Part print with two shaded views. Sizes in mm from the minimum x, y, z corner. A direction names the side the tool comes from. Give positions to 0.01 mm unless a question says otherwise; leave off trailing zeros. Write each loop counter-clockwise with the first axis right and the second up, starting at its lowest first coordinate (ties: lowest second). Pieces come first, ordered by that corner, then holes.
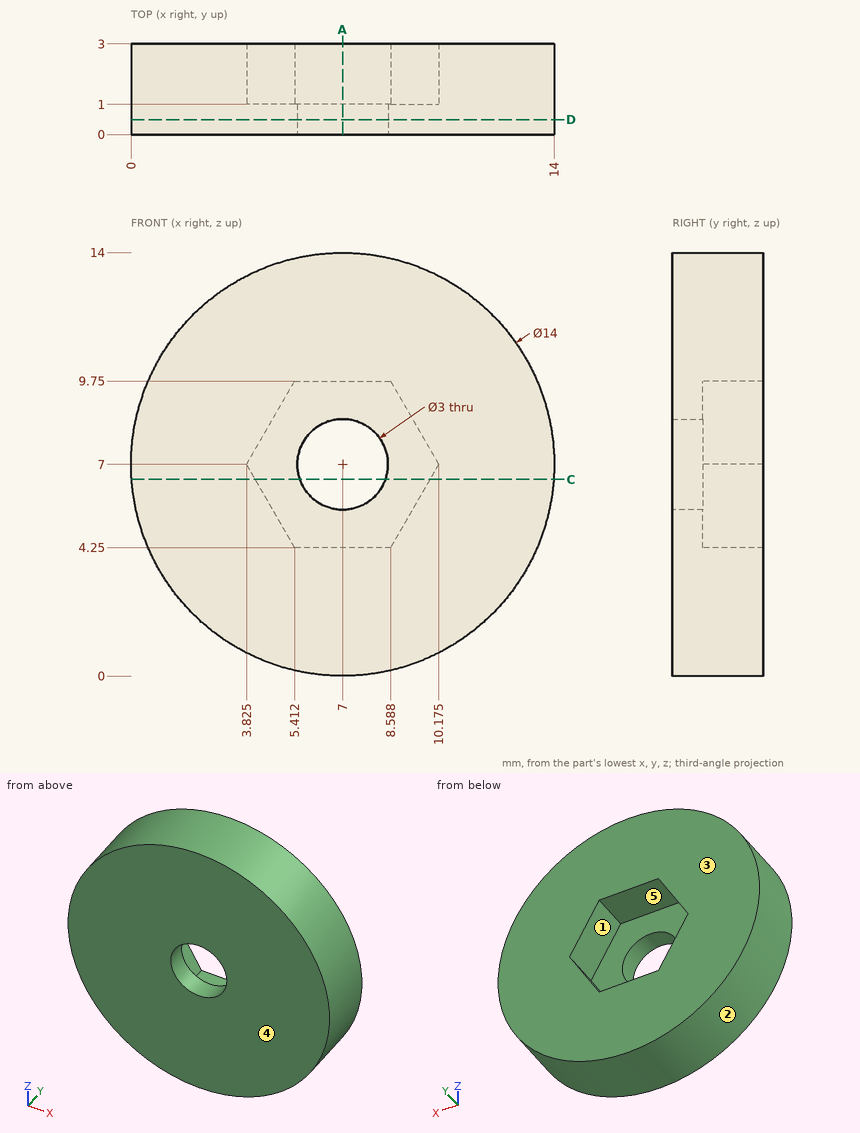
1) 3-axis set-ups, long thin cutter, end or side, ignore diameter. For the marked faces 4 and 5: which of +Z, -Z, +X, -X, +Y, -Y reach the whole face in a straight line?
Answers follow:
face 4: +Z, -Z, +X, -X, -Y
face 5: +Y
2) Saw through at A-A, the plane x = 7. Write the cut outline in (y, z).
Answers follow:
outline: (0, 0) - (3, 0) - (3, 4.25) - (1, 4.25) - (1, 5.5) - (0, 5.5) - close; (0, 8.5) - (1, 8.5) - (1, 9.75) - (3, 9.75) - (3, 14) - (0, 14) - close
3) Pin check, flat tips, straight feed: pin 1 Ø6 at (x, z) = (11, 12.5) entering from -Y; pin 2 Ø3 at (x, z) = (6.5, 6.5) entering from +Y; pin 3 Ø1 at (x, y) = (11.5, 2.5) entering from +Z (1 decimal); pin 4 Ø2.5 at (x, z) = (7, 7) entering from +Y. Stop position of each tip, or through.
Answers follow:
pin 1: stops at y = 0
pin 2: stops at y = 1
pin 3: stops at z = 12.7
pin 4: passes through
4) Two-plate mould, pull along Z, no slides. Class the marked faces 1, 2 and 3: +Z half, -Z half, draft (parallel to the pull), parting line (faces both ways), or undercut.
Answers follow:
face 1: undercut
face 2: parting line
face 3: draft
5) Wall check: L1, parallel to X at y = 0.7, z = 7; L2, parallel to X at y = 2.2, z = 8.5; L3, parallel to Z at x = 5, y = 1.3 (1 decimal). Give the ranges that are in metal, low to high.
Answers follow:
L1: x = 0 to 5.5, 8.5 to 14
L2: x = 0.16 to 4.69, 9.31 to 13.84
L3: z = 0.3 to 5, 9 to 13.7
6) Saw through at C-C, the plane z = 6.5. Write the cut outline in (x, y) (1 decimal).
Answers follow:
outline: (0, 0) - (5.6, 0) - (5.6, 1) - (4.1, 1) - (4.1, 3) - (0, 3) - close; (8.4, 0) - (14, 0) - (14, 3) - (9.9, 3) - (9.9, 1) - (8.4, 1) - close
7) Saw through at D-D, the plane y = 0.5. Write the cut outline in (x, z).
Answers follow:
outline: circle Ø14 at (7, 7); hole circle Ø3 at (7, 7)
